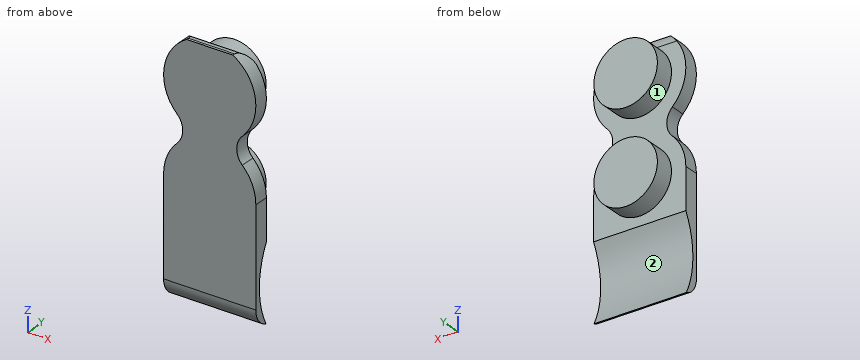
Autodesk Inventor part; units mm, degrees
ref_plane "YZ Plane" through (0, 0, 0) normal (1, 0, 0) x (0, 1, 0)
ref_plane "XZ Plane" through (0, 0, 0) normal (0, 1, 0) x (-1, 0, 0)
ref_plane "XY Plane" through (0, 0, 0) normal (0, 0, 1) x (1, 0, 0)
sketch "Sketch1" plane through (0, 0, 0) normal (0, 1, 0) x (-1, 0, 0)
  line L0 (25.9, 0) -> (-25.9, 0)
  line L1 (0, -25.9) -> (0, 25.9)
  circle A0 centre (0, 0) radius 18.5 construction
  circle A1 centre (0, 0) radius 13 construction
  dimension "d0" = 37
  dimension "d1" = 26
sketch "Sketch2" plane through (0, 0, 0) normal (0, 1, 0) x (-1, 0, 0)
  line L0 (25.9, 0) -> (-25.9, 0)
  line L1 (0, -35.8) -> (0, 67.8)
  line L2 (-18.5, 53) -> (-18.5, -21)
  line L3 (-18.5, -21) -> (18.5, -21)
  line L4 (18.5, -21) -> (18.5, 53)
  line L5 (-18.5, 53) -> (18.5, 53)
  point P0 (0, 0)
  dimension "d3" = 37
  dimension "d29" = 21
  dimension "d30" = 53
extrude "Extrusion1" add sketch "Sketch2" along normal blind 6
sketch "Sketch6" plane through (0, 0, 0) normal (0, 1, 0) x (-1, 0, 0)
  line L0 (18.5, -21) -> (-18.5, -21)
  line L1 (18.5, 53) -> (18.5, -21)
  line L2 (-18.5, -21) -> (18.5, -21)
  line L3 (18.5, -21) -> (18.5, 53)
  line L4 (-18.5, 53) -> (-18.5, -21)
  line L5 (25.9, 0) -> (-25.9, 0)
  line L6 (0, -36.3) -> (0, 70.8)
  arc A0 (-16, 0) -> (16, 0) centre (0, 0) ccw
  line L7 (16, 0) -> (16, 53)
  line L8 (18.5, 53) -> (-18.5, 53)
  line L9 (16, 53) -> (18.5, 53)
  line L10 (-16, 0) -> (-16, 53)
  line L11 (-16, 53) -> (-18.5, 53)
  point P0 (-17.3617, -21)
  dimension "d18" = 32
extrude "Extrusion5" [suppressed]
sketch "Sketch4" plane through (0, 0, 0) normal (0, 0, 1) x (1, 0, 0)
  line L0 (-18.5, 0) -> (18.5, 0)
  line L1 (18.5, 0) -> (18.5, -2)
  line L2 (18.5, -2) -> (-18.5, -2)
  line L3 (-18.5, -2) -> (-18.5, 0)
  line L4 (-25.9, 0) -> (25.9, 0)
  line L5 (0, -2.4) -> (0, 0.4)
  point P0 (0, 0)
  dimension "d10" = 37
  dimension "d11" = 2
extrude "Extrusion6" [suppressed]
sketch "Sketch5" plane through (0, 0, 0) normal (0, 1, 0) x (-1, 0, 0)
  circle A0 centre (0, 0) radius 18.5 construction
  circle A1 centre (0, 0) radius 18.5 construction
  line L0 (25.9, 0) -> (-25.9, 0)
  line L1 (0, -28.9) -> (0, 26.4)
  line L2 (-18.5, -21) -> (18.5, -21)
  line L3 (18.5, -21) -> (18.5, -18.5)
  line L4 (18.5, -18.5) -> (-18.5, -18.5)
  line L5 (-18.5, -18.5) -> (-18.5, -21)
  dimension "d25" = 37
  dimension "d26" = 21
extrude "Extrusion7" [suppressed]
sketch "Sketch7" plane through (0, 0, 0) normal (0, 0, 1) x (1, 0, 0)
  line L0 (-18.5, 0) -> (18.5, 0)
  line L1 (18.5, 0) -> (18.5, -2)
  line L2 (18.5, -2) -> (-18.5, -2)
  line L3 (-18.5, -2) -> (-18.5, 0)
  line L4 (18.5, 0) -> (-18.5, 0)
  line L5 (-25.9, 0) -> (25.9, 0)
  line L6 (0, -2.4) -> (0, 0.4)
  point P0 (-16, 0)
  point P1 (16, 0)
  dimension "d53" = 2
  dimension "d54" = 18.5
extrude "Extrusion8" [suppressed]
sketch "Sketch8" plane through (0, 0, 0) normal (0, 1, 0) x (-1, 0, 0)
  circle A0 centre (0, 0) radius 12.75
  dimension "d34" = 25.5
extrude "Extrusion9" add sketch "Sketch8" along normal blind 14
pattern_linear "Rectangular Pattern1" count 2 spacing 37 along (0, 0, 1) of "Extrusion9"
sketch "Sketch9" plane through (0, 6, 0) normal (0, 1, 0) x (1, 0, 0)
  circle A0 centre (0, 0) radius 13
  circle A1 centre (0, 0) radius 15
  dimension "d40" = 26
  dimension "d41" = 30
extrude "Extrusion10" [suppressed]
sketch "Sketch10" plane through (0, 5, 0) normal (0, 1, 0) x (1, 0, 0)
  arc A0 (16, 0) -> (-16, 0) centre (0, 0) ccw
  line L0 (1.5, -18) -> (-1.5, -18)
  line L1 (-29.4, 0) -> (29.4, 0)
  line L2 (0, 36.3) -> (0, -70.8)
  line L3 (1.5, -12) -> (-1.5, -12)
  line L4 (1.5, -12) -> (1.5, -18)
  line L5 (-1.5, -18) -> (-1.5, -12)
  dimension "d48" = 3
  dimension "d49" = 12
  dimension "d50" = 6
extrude "Extrusion11" [suppressed]
fillet "Fillet1" radius 5 1 edges at (0, 6, 53)
sketch "Sketch11" plane through (0, 0, 0) normal (0, 1, 0) x (-1, 0, 0)
  line L0 (-18.5, -21) -> (18.5, -21)
  line L1 (18.5, -21) -> (18.5, -47)
  line L2 (18.5, -47) -> (-18.5, -47)
  line L3 (-18.5, -47) -> (-18.5, -21)
  line L4 (25.9, 0) -> (-25.9, 0)
  line L5 (0, -60.1) -> (0, 31.6)
  point P0 (0, 0)
  dimension "d57" = 26
  dimension "d58" = 21
  dimension "d59" = 37
extrude "Extrusion12" add sketch "Sketch11" along normal blind 6
sketch "Sketch12" plane through (0, 0, 0) normal (1, 0, 0) x (0, 1, 0)
  line L0 (6, 48) -> (6, -47)
  arc A0 (6, -16.5081) -> (5.7334, -47) centre (34, -32) ccw
  line L1 (-6.8, 0) -> (40.8, 0)
  line L2 (0, -66.5) -> (0, 70)
  line L3 (6, -16.5081) -> (6, -47)
  line L4 (6, -47) -> (5.7334, -47)
  line L5 (0, -47) -> (6, -47)
  point P0 (0, 0)
  dimension "d62" = 32
  dimension "d63" = 32
  dimension "d64" = 34
extrude "Extrusion13" cut sketch "Sketch12" along normal through all both and the other way through all contours L0 L4 A0
fillet "Fillet3" radius 8 1 edges at (0, 0, -47)
sketch "Sketch13" plane through (0, 0, 0) normal (0, 1, 0) x (-1, 0, 0)
  line L0 (25.9, 0) -> (-25.9, 0)
  line L1 (0, -67) -> (0, 73)
  line L2 (18.5, 53) -> (18.5, -39.3278)
  arc A0 (13.0815, 23.9185) -> (13.0815, 13.0815) centre (18.5, 18.5) ccw
  line L3 (-18.5, 48) -> (-18.5, -16.5081)
  arc A1 (-13.0815, 13.0815) -> (-13.0815, 23.9185) centre (-18.5, 18.5) ccw
  line L4 (18.5, 37) -> (18.5, 0)
  line L5 (-18.5, 0) -> (-18.5, 37)
  line L6 (18.5, 37) -> (18.5, 53)
  line L7 (-18.5, 53) -> (18.5, 53)
  line L8 (-18.5, 53) -> (-18.5, 37)
  arc A2 (-9.2871, 53) -> (-13.0815, 23.9185) centre (0, 37) ccw
  arc A3 (13.0815, 23.9185) -> (9.2871, 53) centre (0, 37) ccw
  arc A4 (-13.0815, 13.0815) -> (-18.5, 0) centre (0, 0) ccw
  arc A5 (18.5, 0) -> (13.0815, 13.0815) centre (0, 0) ccw
  dimension "d68" = 37
  dimension "d71" = 18.5
  dimension "d72" = 18.5
  dimension "d73" = 7.663
  dimension "d74" = 7.663
  dimension "d75" = 18.5
  dimension "d76" = 18.5
  dimension "d77" = 18.5
  dimension "d78" = 18.5
extrude "Extrusion14" cut sketch "Sketch13" along normal through all contours A5 A0 A3 L2 | A3 L7 L2 | L3 A2 A1 A4 | L3 L8 L7 A2
properties part number "NespressoSpeedfiller-tamper"
Read the model definition and answer for the solid it produces. Units are mm, in the model's axes. Face numbers are marked on the shaded views. A direction names the side the tool comes from. Coordinates: 2 decimals unless noted, no trailing zeros. Write each loop counter-clockwise with the first axis right and the second up, starting at its lowest first coordinate (ties: lowest second). Pieces come first, ordered by that corner, then holes. Notation, with made-up numbers: (25.25, 88.25) -> (67.25, 88.25) arc R21 ccw to (67.25, 102.25) -> close; hole circle Ø11 at (47.25, -34). An arc over 180 degrees is marked (long way). Answer as a JSON object with one key per item and string values.
Q1. The part is cut by section C-C on y = 10.5. Give the vertices of the cut face in (x, z), then the cut area to 3 significant figures.
The answers:
{"outline": "circle Ø25.5 at (0, 0); circle Ø25.5 at (0, 37)", "area": "1,020 mm2"}
Q2. The part is cut by section D-D on x = -16. Give the vertices of the cut face in (y, z), then the cut area to 3 significant figures.
The answers:
{"outline": "(0, -39.33) arc R8 ccw to (5.73, -47) arc R32 cw to (6, -16.51) -> (6, 9.29) -> (0, 9.29) -> close; (0, 27.71) -> (6, 27.71) -> (6, 46.29) -> (0, 46.29) -> close", "area": "354 mm2"}
Q3. The part is cut by section A-A on z = 37. Give the vertices of the cut face in (x, y), then the cut area to 3 significant figures.
The answers:
{"outline": "(-18.5, 0) -> (18.5, 0) -> (18.5, 6) -> (12.75, 6) -> (12.75, 14) -> (-12.75, 14) -> (-12.75, 6) -> (-18.5, 6) -> close", "area": "426 mm2"}
Q4. Flat-ended cylindrical pins translate along their axes: pin 1 Ø1 at (y, z) = (2.5, 42.5) entering from +X; pin 2 Ø6 at (x, z) = (0, -24.5) entering from +Y; pin 3 Ø2 at (x, y) = (2, 10) entering from -Z. Find the tip coordinate at first contact, or state that the pin passes through.
The answers:
{"pin 1": "stops at x = 17.81", "pin 2": "stops at y = 3.77", "pin 3": "stops at z = -12.71"}
Q5. A tool of negligible diameter and unlimited length cuts with its end or side. For the marked faces 1 and 2, from which of +Z, -Z, +X, -X, +Y, -Y can it reach the whole face along a straight path? Write none if from no direction.
The answers:
{"face 1": "+Y", "face 2": "+X, -X, +Y"}
Q6. The part is cut by section B-B on x = 0. Give the vertices of the cut face in (y, z).
The answers:
{"outline": "(0, -39.33) arc R8 ccw to (5.73, -47) arc R32 cw to (6, -16.51) -> (6, -12.75) -> (14, -12.75) -> (14, 12.75) -> (6, 12.75) -> (6, 24.25) -> (14, 24.25) -> (14, 49.75) -> (5.68, 49.75) arc R5 ccw to (1, 53) -> (0, 53) -> close"}
Q7. Consider line 1 (Y direction, x = 16, z = 34); line 2 (Z direction, x = 10.5, y = 7.25); line 3 (Z direction, x = 6.5, y = 13.5). Determine where each line is inside the solid, lowest interval first. Write a range as [from, to].
The answers:
{"line 1": "y = [0, 6]", "line 2": "z = [-7.23, 7.23], [29.77, 44.23]", "line 3": "z = [-10.97, 10.97], [26.03, 47.97]"}
